Can you work these out from the drawing? Everything is in mm from the part's minimum corner. A direction names the side the tool comes from. Give positions to 0.01 mm unless a question says otherwise; leave off trailing zeros. Write each loop counter-clockwise with the first axis right and the second up, starting at its lowest first coordinate (ties: lowest second). Pieces come first, ordered by that corner, then holes. Notation, with made-up numbers: M 46,35.5 L 92,35.5 A15 cw 92,61.5 Z; hole C 53.5,-13 d6. An arc over 180 degrees is marked long. One line per item, written item: value.
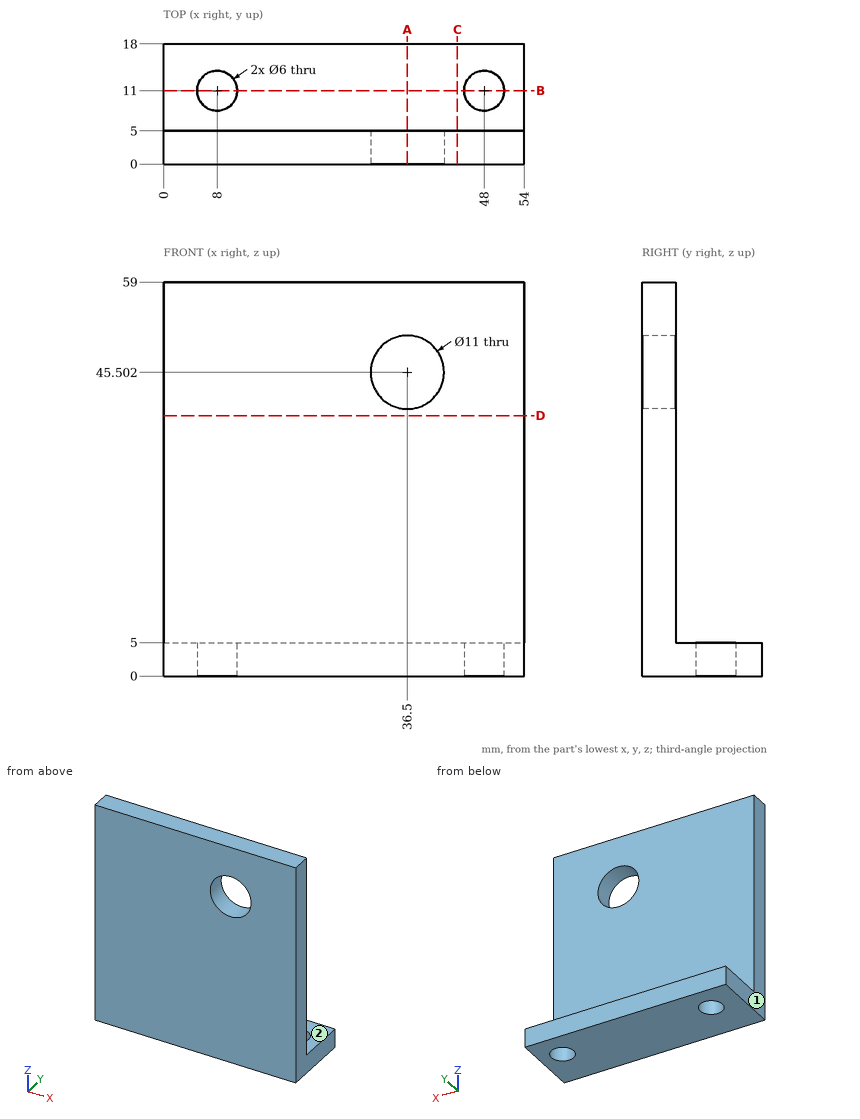
1) If we section it at B-B, the plane y = 11: Write out the boundary of the cut face in (x, z).
Outcome:
outline: M 0,0 L 5,0 L 5,5 L 0,5 Z; M 11,0 L 45,0 L 45,5 L 11,5 Z; M 51,0 L 54,0 L 54,5 L 51,5 Z
2) Please list where these lines run through material, in increasing order: L1, parallel to X at y = 11, z = 1.7; L2, parallel to Y at x = 8, z = 3.75; L3, parallel to Y at x = 11, z = 56. Write a range as from..to.
Outcome:
L1: x = 0..5, 11..45, 51..54
L2: y = 0..8, 14..18
L3: y = 0..5
3) If we section it at A-A, the plane x = 36.5: Write out the boundary of the cut face in (y, z).
Outcome:
outline: M 0,0 L 18,0 L 18,5 L 5,5 L 5,40 L 0,40 Z; M 0,51 L 5,51 L 5,59 L 0,59 Z
4) If we section it at D-D, the plane z = 39: Write out the boundary of the cut face in (x, y).
Outcome:
outline: M 0,0 L 54,0 L 54,5 L 0,5 Z
5) I'm going to push flat-ended pins straight in: pin 1 (10.5 mm diameter, centred on x = 25.5, y = 13.5, fed in from +Z); pin 2 (6 mm diameter, centred on x = 26, z = 23.5, fed in from +Y). Where does each tip first touch, or does it pass through?
Outcome:
pin 1: stops at z = 5
pin 2: stops at y = 5
6) On a 3-axis mill with a long thin cutter (end or side, diameter ignored), from which of +Z, -Z, +X, -X, +Y, -Y can I reach the whole of each face in a straight line? I mean the marked faces 1 and 2. Say none if no direction works.
Outcome:
face 1: +Z, -Z, -X, +Y, -Y
face 2: +Z, +X, -X, +Y
7) If we section it at C-C, the plane x = 44: Write out the boundary of the cut face in (y, z).
Outcome:
outline: M 0,0 L 18,0 L 18,5 L 5,5 L 5,59 L 0,59 Z
